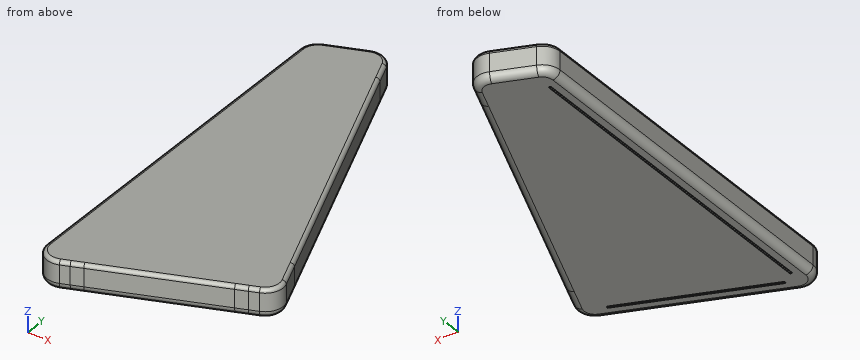
```python
from build123d import *

# Parameters (mm, degrees)
BOSS_EXTRUDE1_DEPTH = 12.7
FILLET1_R           = 3.175
FILLET2_R           = 1.5875
SKETCH3_W           = 0.8128
SKETCH3_H           = 149.86
CUT_EXTRUDE1_DEPTH  = 6.35
CUT_EXTRUDE2_DEPTH  = 6.35


with BuildPart() as part:
    # Sketch1 → Boss-Extrude1 (new body)
    with BuildSketch(Plane.XY):
        with BuildLine():
            Line((73.075190052, 130.577903395), (27.7327817, 247.457923548))
            Line((27.7327817, 247.457923548), (24.400446704, 256.093871545))
            ThreePointArc((24.400446704, 256.093871545), (20.231049001, 260.472170453), (14.186914765, 260.619885912))
            Line((14.186914765, 260.619885912), (-2.107158786, 254.332526198))
            ThreePointArc((-2.107158786, 254.332526198), (-5.777404472, 251.431339634), (-7.1628, 246.962753045))
            Line((-7.1628, 246.962753045), (-7.1628, 243.84))
            Line((-7.1628, 243.84), (-7.1628, 238.76))
            Line((-7.1628, 238.76), (-7.1628, 99.06))
            Line((-7.1628, 99.06), (-7.1628, 93.98))
            Line((-7.1628, 93.98), (-7.1628, 90.008173247))
            ThreePointArc((-7.1628, 90.008173247), (-3.731986589, 83.494168775), (3.580358786, 82.638400094))
            Line((3.580358786, 82.638400094), (7.285888595, 84.068245047))
            Line((7.285888595, 84.068245047), (12.025292552, 85.897028832))
            Line((12.025292552, 85.897028832), (64.158736078, 106.01365047))
            Line((64.158736078, 106.01365047), (68.898140035, 107.842434255))
            Line((68.898140035, 107.842434255), (72.80002218, 109.34804527))
            ThreePointArc((72.80002218, 109.34804527), (77.178321088, 113.517442972), (77.326036547, 119.561577209))
            Line((77.326036547, 119.561577209), (73.075190052, 130.577903395))
        make_face()
    extrude(amount=BOSS_EXTRUDE1_DEPTH)

    # Fillet1
    fillet1_edges = [part.edges().sort_by_distance(p)[0] for p in [
        (-7.1628, 168.485463146, 0),
        (-3.731986589, 83.494168775, 0),
        (38.190190483, 95.993222682, 0),
        (77.178321088, 113.517442972, 0),
        (75.200613299, 125.069740302, 0),
        (50.403985876, 189.017913472, 0),
        (26.066614202, 251.775897547, 0),
        (20.231049001, 260.472170453, 0),
        (6.039877989, 257.476206055, 0),
        (-5.777404472, 251.431339634, 0),
    ]]
    fillet(fillet1_edges, radius=FILLET1_R)

    # Fillet2
    fillet2_edges = [part.edges().sort_by_distance(p)[0] for p in [
        (-5.777404472, 251.431339634, 12.7),
        (6.039877989, 257.476206055, 12.7),
        (20.231049001, 260.472170453, 12.7),
        (26.066614202, 251.775897547, 12.7),
        (50.403985876, 189.017913472, 12.7),
        (75.200613299, 125.069740302, 12.7),
        (77.178321088, 113.517442972, 12.7),
        (38.190190483, 95.993222682, 12.7),
        (-7.1628, 168.485463146, 12.7),
        (-3.731986589, 83.494168775, 12.7),
    ]]
    fillet(fillet2_edges, radius=FILLET2_R)

    # Sketch3 → Cut-Extrude1 (cut)
    with BuildSketch(Plane(origin=(0, 0, 0), x_dir=(-1, 0, 0), z_dir=(0, 0, -1))):
        with Locations((0.4064, 168.91)):
            Rectangle(SKETCH3_W, SKETCH3_H)
    extrude(amount=-CUT_EXTRUDE1_DEPTH, mode=Mode.SUBTRACT)

    # Sketch4 → Cut-Extrude2 (cut)
    with BuildSketch(Plane(origin=(0, 0, 0), x_dir=(-1, 0, 0), z_dir=(0, 0, -1))):
        Polygon((-66.319554898, 114.524993835), (-4.707303458, 90.750804626), (-4.999908864, 89.992499993), (-66.612160304, 113.766689202), align=None)
    extrude(amount=-CUT_EXTRUDE2_DEPTH, mode=Mode.SUBTRACT)


solid = part.part
```
Here's how the part is built. I have some questions about the finished solid (model axes, mm). Give positions to 0.01 mm unless a question says otherwise; leave off trailing zeros. Order: outer loops, then holes, each group sorted by start corner. A loop starts at its lowest first (then second) coordinate and runs counter-clockwise, first axis right, second up. Notation, with made-up numbers: M 16.5,32 L 21.5,32 A24 cw 21.5,52 Z; hole C 61,23.5 d8. An arc over 180 degrees is marked long. Use a Markdown table: item, result. Add a question column.
1. For pin 1 Ø6 at (x, z) = (4.5, 6.5) entering from +Y; pin 2 Ø0.9 at (x, y) = (-0.5, 137.5) entering from -Z; pin 3 Ø5 at (y, z) = (192.5, 3.5) entering from +X; pin 4 Ø0.9 at (x, z) = (-0.5, 4.5) entering from +Y, each with a flat end and sliding along its axis, tell me the tip position at first contact or that it passes through.
2. Suppose I cut it at A-A (z = 8.75). List the corners of the cut face in (x, y) for me.
3. I need wall thicknesses on probe 1 along X at (y, z) = (239, 3.25); probe 2 along X at (y, z) = (190, 3.25); probe 3 along X at (y, z) = (250.5, 11.75). Which ranges of each line are inside material? Lowest first, please. Write a range as from..to.
Results list:
| question | item | result |
|---|---|---|
| 1 | pin 1 | stops at y = 258.04 |
| 1 | pin 2 | stops at z = 0 |
| 1 | pin 3 | stops at x = 50.02 |
| 1 | pin 4 | stops at y = 255.13 |
| 2 | outline | M -7.16,90.01 A7.9 ccw 3.58,82.64 L 72.8,109.35 A7.9 ccw 77.33,119.56 L 73.08,130.58 L 27.73,247.46 L 24.4,256.09 A7.9 ccw 14.19,260.62 L -2.11,254.33 A7.9 ccw -7.16,246.96 Z |
| 3 | probe 1 | x = -7.16..-0.81, 0..31.01 |
| 3 | probe 2 | x = -7.16..-0.81, 0..50.02 |
| 3 | probe 3 | x = -6.18..26.42 |
